Could you check a few things on this model? Use its own coordinates, in mm. Coordinates: 2 decimals unless noted, no trailing zeros. Write each loop counter-clockwise with the first axis right and the second up, starting at its lowest first coordinate (ties: lowest second). Pieces come first, ordered by that corner, then holes.
```python
from build123d import *

# Parameters (mm, degrees)
SKETCH1_W           = 92.44
SKETCH1_H           = 53
BOSS_EXTRUDE1_DEPTH = 2
SKETCH2_R           = 1.5
CUT_EXTRUDE1_DEPTH  = 3
SKETCH3_R           = 2.5
SKETCH3_W           = 32
SKETCH3_H           = 35
SKETCH3_W_2         = 14.2
SKETCH3_H_2         = 7
SKETCH3_W_3         = 12.6
SKETCH3_H_3         = 19.5
CUT_EXTRUDE2_DEPTH  = 3


with BuildPart() as part:
    # Sketch1 → Boss-Extrude1 (new body)
    with BuildSketch(Plane(origin=(0, 0, 0), x_dir=(1, 0, 0), z_dir=(0, 1, 0))):
        Rectangle(SKETCH1_W, SKETCH1_H)
    extrude(amount=BOSS_EXTRUDE1_DEPTH)

    # Sketch2 → Cut-Extrude1 (cut, through all)
    with BuildSketch(Plane(origin=(0, 2, 0), x_dir=(1, 0, 0), z_dir=(0, 1, 0))):
        with Locations((-43.72, 24)):
            Circle(SKETCH2_R)
        with Locations((43.72, 24)):
            Circle(SKETCH2_R)
        with Locations((43.72, -24)):
            Circle(SKETCH2_R)
        with Locations((-43.72, -24)):
            Circle(SKETCH2_R)
    extrude(amount=-CUT_EXTRUDE1_DEPTH, mode=Mode.SUBTRACT)

    # Sketch3 → Cut-Extrude2 (cut, through all)
    with BuildSketch(Plane(origin=(0, 2, 0), x_dir=(1, 0, 0), z_dir=(0, 1, 0))):
        with Locations((38.58, 5)):
            Circle(SKETCH3_R)
        with Locations((-20.22, 1.5)):
            Rectangle(SKETCH3_W, SKETCH3_H)
        with Locations((7.88, 15.5)):
            Rectangle(SKETCH3_W_2, SKETCH3_H_2)
        with Locations((27.08, 15.5)):
            Rectangle(SKETCH3_W_2, SKETCH3_H_2)
        with Locations((7.08, -2.75)):
            Rectangle(SKETCH3_W_3, SKETCH3_H_3)
        with Locations((26.28, -2.75)):
            Rectangle(SKETCH3_W_3, SKETCH3_H_3)
    extrude(amount=-CUT_EXTRUDE2_DEPTH, mode=Mode.SUBTRACT)


solid = part.part
```
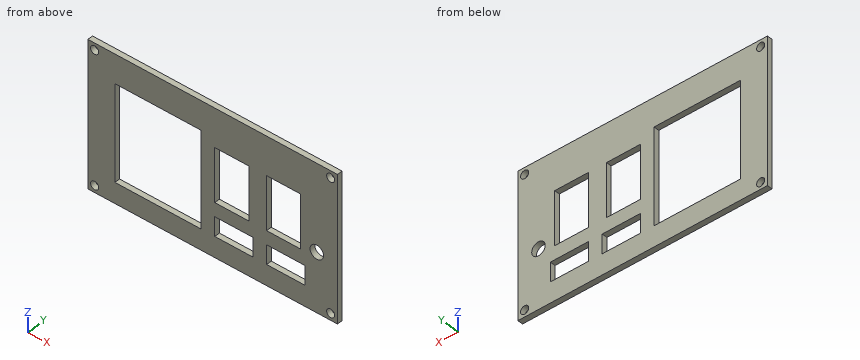
1. I want a section at C-C on z = -5. Please give me the cut outline in (x, y), plus the area to 3 significant figures.
Verdict:
outline: (-46.22, 0) - (-36.22, 0) - (-36.22, 2) - (-46.22, 2) - close; (-4.22, 0) - (0.78, 0) - (0.78, 2) - (-4.22, 2) - close; (13.38, 0) - (19.98, 0) - (19.98, 2) - (13.38, 2) - close; (32.58, 0) - (36.08, 0) - (36.08, 2) - (32.58, 2) - close; (41.08, 0) - (46.22, 0) - (46.22, 2) - (41.08, 2) - close
area: 60.5 mm2
2. Please list where these lines run through material, in increasing order: line 1 along X through (y, z) = (0.25, 8.5); line 2 along Z through (x, y) = (-43.72, 0.85); line 3 along Z through (x, y) = (2.5, 1.45).
Verdict:
line 1: x = -46.22 to -36.22, -4.22 to 0.78, 13.38 to 19.98, 32.58 to 46.22
line 2: z = -26.5 to -25.5, -22.5 to 22.5, 25.5 to 26.5
line 3: z = -26.5 to -19, -12 to -7, 12.5 to 26.5
3. I want a section at A-A on z = 24. Please give me the cut outline in (x, y).
Verdict:
outline: (-46.22, 0) - (-45.22, 0) - (-45.22, 2) - (-46.22, 2) - close; (-42.22, 0) - (42.22, 0) - (42.22, 2) - (-42.22, 2) - close; (45.22, 0) - (46.22, 0) - (46.22, 2) - (45.22, 2) - close
4. I want a section at D-D on y = 0.9. Give the number of separate pieces and of enclosed holes in the cut face, plus the area to 3 significant figures.
Verdict:
separate pieces: 1
enclosed holes: 10
area: 3,040 mm2
5. I want a section at B-B on x = 38.58. Please give me the cut outline in (y, z).
Verdict:
outline: (0, -26.5) - (2, -26.5) - (2, -7.5) - (0, -7.5) - close; (0, -2.5) - (2, -2.5) - (2, 26.5) - (0, 26.5) - close
6. For pin 1 (12 mm diameter, centred on x = -5.5, z = 14, fed in from -Y), with a flat end and sliding along its axis, tell me the tip position at first contact or that it passes through.
Verdict:
pin 1: stops at y = 0
